The listing builds one solid part. Answer for the finished solid, in the listing's coordinates (mm). Face numbers are marked on the shaded views. A direction names the side the tool comes from. Round coordinates to 2 decimals unless told otherwise and drop trailing zeros. Write each loop counter-clockwise with the first axis right and the second up, starting at its lowest first coordinate (ties: lowest second). Pieces come first, ordered by that corner, then holes.
Item 1: Find section D-D on y = 40.5. Give the vertices of the cut face in (x, z), then the cut area to 3 significant figures.
Item 2: A tool of negligible diameter and unlimited length cuts with its end or side. For the marked faces 1 and 2, from which of +Z, -Z, +X, -X, +Y, -Y can it reach the whole face along a straight path? Write none if from no direction.
Item 3: Find the intervals of material crossed by probe 1 along Z at (x, y) = (1.25, 53); probe 2 along Y at (x, z) = (2.5, 4.5); probe 3 along X at (y, z) = (42.5, 3.5), in increasing order.
Item 4: Find section C-C on z = 2. Give the vertices of the cut face in (x, y), then the cut area to 3 significant figures.
Item 5: This flat-tipped pin is pushed along its axis until it touches: pin 1 (2.5 mm diameter, centred on y = 41.5, z = 6.5, fed in from +X). Where does it stop, or does it pass through?
Item 6: Find section A-A on z = 4.5. Give the vertices of the cut face in (x, y).
Item 7: Find section B-B on x = 0.75. Give the vertices of the cut face in (y, z), then the cut area to 3 significant figures.
```python
from build123d import *

# Parameters (mm, degrees)
EXTRUDE_1_DEPTH     = 9
CUT_EXTRUDE_2_DEPTH = 68.284842275
EXTRUDE_2_DEPTH     = 9


with BuildPart() as part:
    # Эскиз1 → Бобышка-Вытянуть1 (new body)
    with BuildSketch(Plane.XY):
        Polygon((0, 0), (9.5, 0), (9.5, 3), (3, 3), (3, 66), (0, 66), align=None)
    extrude(amount=EXTRUDE_1_DEPTH)

    # Эскиз4 → Вырез-Вытянуть2 (cut, through all)
    with BuildSketch(Plane.ZY):
        with BuildLine():
            Line((6.25, 55.52), (6.25, 49.52))
            ThreePointArc((6.25, 49.52), (4.5, 47.77), (2.75, 49.52))
            Line((2.75, 49.52), (2.75, 55.52))
            ThreePointArc((2.75, 55.52), (4.5, 57.27), (6.25, 55.52))
        make_face()
    extrude(amount=-CUT_EXTRUDE_2_DEPTH, mode=Mode.SUBTRACT)

    # Эскиз5 → Бобышка-Вытянуть2 (add, through all)
    with BuildSketch(Plane.XY.offset(9)):
        Polygon((3, 3), (3, 10), (9.5, 3), align=None)
    extrude(amount=-EXTRUDE_2_DEPTH)


solid = part.part
```
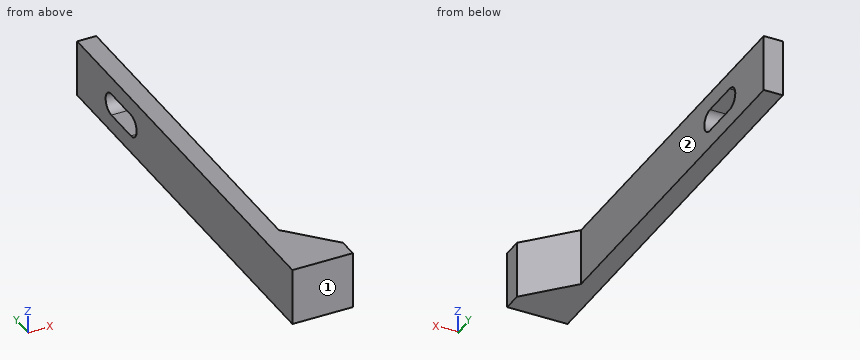
Check values:
1. outline: (0, 0) - (3, 0) - (3, 9) - (0, 9) - close
1. area: 27.0 mm2
2. face 1: +Z, -Z, +X, -X, -Y
2. face 2: +Z, -Z, +X, +Y
3. probe 1: z = 0 to 2.75, 6.25 to 9
3. probe 2: y = 0 to 47.77, 57.27 to 66
3. probe 3: x = 0 to 3
4. outline: (0, 0) - (9.5, 0) - (9.5, 3) - (3, 10) - (3, 66) - (0, 66) - close
4. area: 240 mm2
5. pin 1: stops at x = 3
6. outline: (0, 0) - (9.5, 0) - (9.5, 3) - (3, 10) - (3, 47.77) - (0, 47.77) - close; (0, 57.27) - (3, 57.27) - (3, 66) - (0, 66) - close
7. outline: (0, 0) - (66, 0) - (66, 9) - (0, 9) - close; hole (49.52, 2.75) - (55.52, 2.75) arc R1.75 ccw to (55.52, 6.25) - (49.52, 6.25) arc R1.75 ccw to start
7. area: 563 mm2
